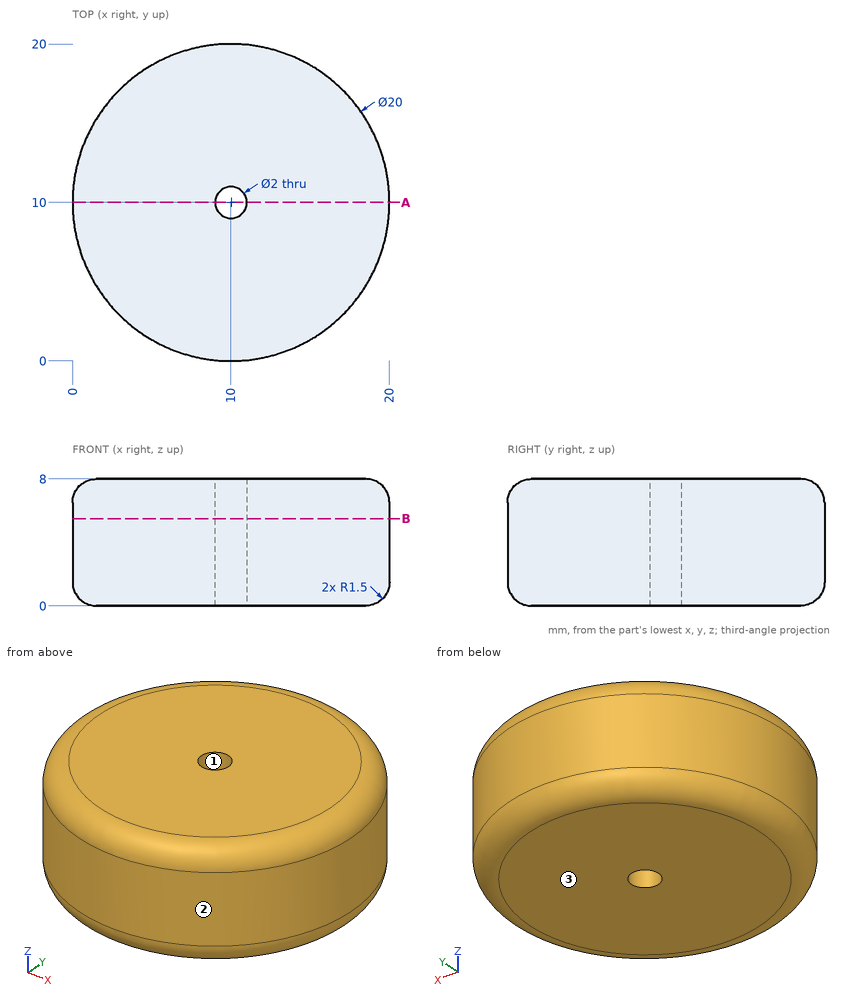
Can you work these out from the drawing? Everything is in mm from the part's minimum corner. Give positions to 0.01 mm unless a question says otherwise; leave off trailing zeros. Order: outer loops, then holes, each group sorted by start corner. A loop starts at its lowest first (then second) coordinate and runs counter-clockwise, first axis right, second up. Notation, with made-up numbers: M 45.5,30 L 64.5,30 A22 ccw 64.5,40 Z; hole C -31,23 d5. An arc over 180 degrees is marked long. Use a Markdown table: item, result. Add a question column.
1. If we mould it in two halves opening along X, with no side actions, what happens to the marked faces 1, 2 and 3? For each: +X half, -X half, draft (parallel to the pull), parting line (faces both ways), or undercut.
2. Suppose I cut it at A-A (y = 10). List the corners of the cut face in (x, z) for me, and give its area (3 significant figures).
3. Suppose I cut it at B-B (z = 5.5). List the corners of the cut face in (x, y) for me, and give its area (3 significant figures).
4. I need wall thicknesses on probe 1 along Y at (x, z) = (10, 3.5); probe 2 along Y at (x, z) = (2, 3); probe 3 along Z at (x, y) = (18, 5.75). Which ranges of each line are inside material? Lowest first, please. Write a range as from..to.
5. For pin 1 Ø1 at (x, z) = (16.5, 3) entering from -Y; pin 2 Ø1.6 at (x, y) = (10, 10) entering from -Z; pin 3 Ø2 at (y, z) = (4.5, 5) entering from +X, each with a flat end and sliding along its axis, tell me the tip position at first contact or that it passes through.
Results list:
| question | item | result |
|---|---|---|
| 1 | face 1 | undercut |
| 1 | face 2 | parting line |
| 1 | face 3 | draft |
| 2 | outline | M 0,1.5 A1.5 ccw 1.5,0 L 9,0 L 9,8 L 1.5,8 A1.5 ccw 0,6.5 Z; M 11,0 L 18.5,0 A1.5 ccw 20,1.5 L 20,6.5 A1.5 ccw 18.5,8 L 11,8 Z |
| 2 | area | 142 mm² |
| 3 | outline | C 10,10 d20; hole C 10,10 d2 |
| 3 | area | 311 mm² |
| 4 | probe 1 | y = 0..9, 11..20 |
| 4 | probe 2 | y = 4..16 |
| 4 | probe 3 | z = 0.11..7.89 |
| 5 | pin 1 | stops at y = 2 |
| 5 | pin 2 | passes through |
| 5 | pin 3 | stops at x = 18.93 |
